```python
from build123d import *

# Parameters (mm, degrees)
SKETCH3_W                = 15
SKETCH3_H                = 16
BOSS_EXTRUDE1_DEPTH      = 2.5
SKETCH4_W                = 2.5
SKETCH4_H                = 16
BOSS_EXTRUDE2_DEPTH      = 9.8
M2_CLEARANCE_HOLE1_D     = 2.4
M2_CLEARANCE_HOLE1_DEPTH = 15
M2_CLEARANCE_HOLE1_TIP   = 0.721032743
FILLET1_R                = 2
BOSS_EXTRUDE3_START      = 4
SKETCH9_W                = 16
SKETCH9_H                = 6
SKETCH9_R                = 1.2
BOSS_EXTRUDE3_DEPTH      = 4
FILLET2_R                = 2
CUT_EXTRUDE1_START       = -1.25
CUT_EXTRUDE1_DEPTH       = 2


with BuildPart() as part:
    # Sketch3 → Boss-Extrude1 (new body)
    with BuildSketch(Plane(origin=(0, 0, 0), x_dir=(1, 0, 0), z_dir=(0, 1, 0))):
        Rectangle(SKETCH3_W, SKETCH3_H)
    extrude(amount=BOSS_EXTRUDE1_DEPTH)

    # Sketch4 → Boss-Extrude2 (add)
    with BuildSketch(Plane(origin=(0, 2.5, 0), x_dir=(1, 0, 0), z_dir=(0, 1, 0))):
        with Locations((-6.25, 0)):
            Rectangle(SKETCH4_W, SKETCH4_H)
        with Locations((6.25, 0)):
            Rectangle(SKETCH4_W, SKETCH4_H)
    extrude(amount=BOSS_EXTRUDE2_DEPTH)

    # M2 Clearance Hole1
    with Locations(Plane(origin=(7.5, 0, 0), x_dir=(0, 0, -1), z_dir=(1, 0, 0))):
        with Locations((-4, 9.3), (4, 9.3)):
            Hole(M2_CLEARANCE_HOLE1_D / 2, depth=M2_CLEARANCE_HOLE1_DEPTH)
            with Locations((0, 0, -(M2_CLEARANCE_HOLE1_DEPTH + M2_CLEARANCE_HOLE1_TIP / 2))):  # 118° drill point
                Cone(0, M2_CLEARANCE_HOLE1_D / 2, M2_CLEARANCE_HOLE1_TIP, mode=Mode.SUBTRACT)

    # Fillet1
    fillet1_edges = [part.edges().sort_by_distance(p)[0] for p in [
        (-7.5, 0, 0),
        (7.5, 0, 0),
    ]]
    fillet(fillet1_edges, radius=FILLET1_R)

    # Sketch9 → Boss-Extrude3 (add)
    with BuildSketch(Plane.ZY.offset(-5).offset(BOSS_EXTRUDE3_START)):
        with Locations((0, 9.3)):
            Rectangle(SKETCH9_W, SKETCH9_H)
        with Locations(Location((-4, 9.3, 0), (0, 0, 180))):
            Circle(SKETCH9_R, mode=Mode.SUBTRACT)
        with Locations(Location((4, 9.3, 0), (0, 0, 180))):
            Circle(SKETCH9_R, mode=Mode.SUBTRACT)
    extrude(amount=-BOSS_EXTRUDE3_DEPTH)

    # Fillet2
    # the kernel refuses this fillet: 2 mm, written as the material it takes off along each edge
    with BuildSketch(Plane(origin=(-7.5, 12.3, 13), x_dir=(1, 0, 0), z_dir=(0, 0, -1)), Plane(origin=(1, 6.3, 13), x_dir=(0, 1, 0), z_dir=(0, 0, -1))) as fillet2_piece_1:
        with BuildLine():
            CenterArc((FILLET2_R, FILLET2_R), FILLET2_R, 180, 90)
            Line((0, FILLET2_R), (0, 0))
            Line((0, 0), (FILLET2_R, 0))
        make_face()
    extrude(amount=26, mode=Mode.SUBTRACT)
    with BuildSketch(Plane(origin=(7.5, 12.3, -13), x_dir=(0, -1, 0), z_dir=(0, 0, 1))) as fillet2_piece_2:
        with BuildLine():
            CenterArc((FILLET2_R, -FILLET2_R), FILLET2_R, 90, 90)
            Line((0, -FILLET2_R), (0, 0))
            Line((0, 0), (FILLET2_R, 0))
        make_face()
    extrude(amount=26, mode=Mode.SUBTRACT)

    # Sketch10 → Cut-Extrude1 (cut)
    with BuildSketch(Plane(origin=(7.5, 0, 0), x_dir=(0, 0, -1), z_dir=(1, 0, 0)).offset(CUT_EXTRUDE1_START)):
        Polygon((-4, 6.817393842), (-1.85, 8.058696921), (-1.85, 10.541303079), (-1.85, 12.3), (-6.15, 12.3), (-6.15, 10.541303079), (-6.15, 8.058696921), align=None)
        Polygon((4, 6.817393842), (6.15, 8.058696921), (6.15, 10.541303079), (6.15, 12.3), (1.85, 12.3), (1.85, 10.541303079), (1.85, 8.058696921), align=None)
    extrude(amount=-CUT_EXTRUDE1_DEPTH, mode=Mode.SUBTRACT)


solid = part.part
```
Geometry check sheet. Reference: the model listing, model coordinates, mm. A direction names the side the tool comes from. Coordinates: 2 decimals unless noted, no trailing zeros. Order: outer loops, then holes, each group sorted by start corner. A loop starts at its lowest first (then second) coordinate and runs counter-clockwise, first axis right, second up.
Q1. Depth check by flat-ended pin: pin 1 Ø2 at (y, z) = (8.5, -4.5) entering from -X. Enter the tip coordinate at first touch or a pass-through.
Reply:
pin 1: stops at x = -7.5
Q2. Sectioned sample at C-C on x = 5.75. Record the cut outline in (y, z).
Reply:
outline: (0.02, -8) - (12.28, -8) - (12.28, -6.15) - (8.06, -6.15) - (6.82, -4) - (8.06, -1.85) - (12.28, -1.85) - (12.28, 1.85) - (8.06, 1.85) - (6.82, 4) - (8.06, 6.15) - (12.28, 6.15) - (12.28, 8) - (0.02, 8) - close
Q3. Sectioned sample at D-D on y = 9.3. Give the number of separate pieces and of enclosed holes in the cut face, and give its area (3 significant figures).
Reply:
separate pieces: 6
enclosed holes: 0
area: 93.2 mm2
Q4. Draft check along X on faces 4 (the face through (2, 7, 8)), 5 (the face through (5.264, 7.447, 5.09)), 6 (the face through (6.25, 11, 4)), 7 (the face through (-6.93, 0.6, -0.11)). Enter one of: released by +X, released by -X, zero draft, split by the parting line, or undercut.
Reply:
face 4: zero draft
face 5: undercut
face 6: undercut
face 7: released by -X
Q5. Sectioned sample at A-A on y = 5.5. Record the cut outline in (x, z).
Reply:
outline: (-7.5, -8) - (-5, -8) - (-5, 8) - (-7.5, 8) - close; (5, -8) - (7.5, -8) - (7.5, 8) - (5, 8) - close
Q6. Sectioned sample at B-B on z = -1.25. Record the cut outline in (x, y).
Reply:
outline: (-7.5, 2) arc R2 ccw to (-5.5, 0) - (5.5, 0) arc R2 ccw to (7.5, 2) - (7.5, 10.3) arc R2 ccw to (5.5, 12.3) - (1, 12.3) - (1, 8.3) arc R2 ccw to (3, 6.3) - (5, 6.3) - (5, 2.5) - (-5, 2.5) - (-5, 12.3) - (-5.5, 12.3) arc R2 ccw to (-7.5, 10.3) - close
Q7. Tool access check on faces 1 (the face through (5, 4, 0)), 2 (the face through (6.25, 11, -4)), 3 (the face through (2.6, 10.47, -3.74)). Record the directions out of +Z, -Z, +X, -X, +Y, -Y that give a thin tool (end or side, any length) a straight path to the whole face; none if there is none.
Reply:
face 1: +Z, -Z
face 2: +Y
face 3: +X, -X
Q8. Thickness scan on probe 1 along Z at (x, y) = (-6.5, 9.3); probe 2 along X at (y, z) = (5.5, -3); probe 3 along Y at (x, z) = (2.65, 4). Record the ranges inside material, lowest first.
Reply:
probe 1: z = -8 to -5.2, -2.8 to 2.8, 5.2 to 8
probe 2: x = -7.5 to -5, 5 to 7.5
probe 3: y = 0 to 2.5, 6.33 to 8.1, 10.5 to 12.3
